Autodesk Fusion 360 part; units mm, degrees
sketch "Sketch1" plane through (0, 0, 0) normal (0, 1, 0) x (1, 0, 0)
  line L0 (0, 0) -> (60, 0)
  line L1 (60, 0) -> (60, 44)
  line L2 (60, 44) -> (0, 44)
  line L3 (0, 44) -> (0, 0)
  line L4 (3, 41) -> (57, 41)
  line L5 (57, 41) -> (57, 3)
  line L6 (57, 3) -> (3, 3)
  line L7 (3, 3) -> (3, 41)
  circle A0 centre (7, 37) radius 1.6
  circle A1 centre (53, 37) radius 1.6
  line L8 (3, 22) -> (57, 22)
  circle A2 centre (7, 7) radius 1.6
  circle A3 centre (53, 7) radius 1.6
  dimension "d1" = 60
  dimension "d2" = 44
  dimension "d3" = 54
  dimension "d4" = 38
  dimension "d9" = 3.2
  dimension "d10" = 3.2
extrude "Extrude1" add sketch "Sketch1" against normal blind 2 contours L0 L1 L2 L3 | L4 L5 L7 L8 | L5 L6 L7 L8 | A0 | A1 | A2 | A3
extrude "Extrude2" add sketch "Sketch1" along normal blind 2 contours L4 L5 L7 L8 | L5 L6 L7 L8 | A0 | A1 | A2 | A3
extrude "Extrude3" cut sketch "Sketch1" along normal blind 3 contours A0 | A1 | A2 | A3
extrude "Extrude4" cut sketch "Sketch1" against normal blind 8 contours A0 | A1 | A2 | A3
chamfer "Chamfer1" distance 0.75 angle 45 4 edges at (5.5083, -2, -6.4214) (5.5083, -2, -36.4214) (51.5083, -2, -36.4214) (51.5083, -2, -6.4214)
delete_face "DeleteFace1" 1 faces at (54.892, -1.75, -6.0888)
delete_face "DeleteFace2" 1 faces at (54.892, -1.75, -36.0888)
delete_face "DeleteFace3" 1 faces at (8.05, -1.75, -8.8187)
delete_face "DeleteFace4" 1 faces at (5.2649, -1.75, -38.183)
chamfer "Chamfer2" distance 1.5 angle 45 4 edges at (5.5083, -2, -7.5786) (51.5083, -2, -7.5786) (51.5083, -2, -37.5786) (5.5083, -2, -37.5786)
equation "d3 = 118 mm - 64 mm"
Can you work these out from the model? Positions are in its coordinate system, mm. A direction names the side the tool comes from. Coordinates: 2 decimals unless noted, no trailing zeros. Write each loop counter-clockwise with the first axis right and the second up, starting at its lowest first coordinate (ties: lowest second). Pieces come first, ordered by that corner, then holes. Notation, with made-up numbers: (-5, -31.5) - (3, -31.5) arc R26 ccw to (3, -9.5) - close; hole circle Ø2 at (52, -21). An arc over 180 degrees is marked (long way). Return JSON: item names as keys, results as strings. Group by question number.
Item 1: We'd pull the mould along X, two halves only. Please class faces 4 (the face through (54.48, 0.77, -6.39)), 5 (the face through (3, 1, -22)), 6 (the face through (30, -2, -22)): pulls with the +X half, pulls with the -X half, needs draft (parallel to the pull), parting line crosses it, or undercut.
Item 2: If we section it at B-B (x = 53): Write out the boundary of the cut face in (y, z).
Item 3: I'm going to push flat-ended pins straight in: pin 1 Ø1 at (y, z) = (1.5, -14) entering from -X; pin 2 Ø3.5 at (x, z) = (53, -7) entering from -Y; pin 3 Ø1 at (x, y) = (33, 1.5) entering from +Z. Where does each tip first touch, or does it pass through?
Item 4: If we section it at D-D (x = 24): Write out the boundary of the cut face in (y, z), then the cut area to 3 significant figures.
Item 5: If we section it at A-A (z = -37): Write out the boundary of the cut face in (x, y), then the cut area to 3 significant figures.
Item 6: Please list where these lines run through material, in increasing order: probe 1 along Z at (x, y) = (53, 0.5); probe 2 along X at (y, z) = (1.1, -7); probe 3 along X at (y, z) = (-1.3, -7.5).
Item 7: If we section it at C-C (y = 0.95): Write out the boundary of the cut face in (x, z), then the cut area to 3 significant figures.
Item 8: Which directions (+Z, -Z, +X, -X, +Y, -Y) give clear straight access to the entire face, cutting with the end or side of a thin tool? Please do faces 1 (the face through (57, 1, -22)), 2 (the face through (30, 1, -41)), 3 (the face through (30, 1, -3)).
Return value:
{
 "1": {"face 4": "undercut", "face 5": "pulls with the -X half", "face 6": "needs draft"},
 "2": {"outline": "(-2, -44) - (0, -44) - (0, -41) - (2, -41) - (2, -38.6) - (-0.5, -38.6) - (-2, -40.1) - close; (-2, -33.9) - (-0.5, -35.4) - (2, -35.4) - (2, -8.6) - (-0.5, -8.6) - (-2, -10.1) - close; (-2, -3.9) - (-0.5, -5.4) - (2, -5.4) - (2, -3) - (0, -3) - (0, 0) - (-2, 0) - close"},
 "3": {"pin 1": "stops at x = 3", "pin 2": "stops at y = -0.65", "pin 3": "stops at z = -3"},
 "4": {"outline": "(-2, -44) - (0, -44) - (0, -41) - (2, -41) - (2, -3) - (0, -3) - (0, 0) - (-2, 0) - close", "area": "164 mm^2"},
 "5": {"outline": "(0, -2) - (3.9, -2) - (5.4, -0.5) - (5.4, 2) - (3, 2) - (3, 0) - (0, 0) - close; (8.6, -0.5) - (10.1, -2) - (49.9, -2) - (51.4, -0.5) - (51.4, 2) - (8.6, 2) - close; (54.6, -0.5) - (56.1, -2) - (60, -2) - (60, 0) - (57, 0) - (57, 2) - (54.6, 2) - close", "area": "198 mm^2"},
 "6": {"probe 1": "z = -41 to -38.6, -35.4 to -8.6, -5.4 to -3", "probe 2": "x = 3 to 5.4, 8.6 to 51.4, 54.6 to 57", "probe 3": "x = 0 to 4.65, 9.35 to 50.65, 55.35 to 60"},
 "7": {"outline": "(3, -41) - (57, -41) - (57, -3) - (3, -3) - close; hole circle Ø3.2 at (7, -37); hole circle Ø3.2 at (7, -7); hole circle Ø3.2 at (53, -37); hole circle Ø3.2 at (53, -7)", "area": "2,020 mm^2"},
 "8": {"face 1": "+Z, -Z, +X, +Y", "face 2": "-Z, +X, -X, +Y", "face 3": "+Z, +X, -X, +Y"}
}
